Autodesk Fusion 360 part; units mm, degrees
sketch "Sketch1" plane through (0, 0, 0) normal (0, 1, 0) x (1, 0, 0)
  line L0 (1.775, -3.0744) -> (3.55, 0)
  line L1 (3.55, 0) -> (1.775, 3.0744)
  line L2 (1.775, 3.0744) -> (-1.775, 3.0744)
  line L3 (-1.775, 3.0744) -> (-3.55, 0)
  line L4 (-3.55, 0) -> (-1.775, -3.0744)
  line L5 (-1.775, -3.0744) -> (1.775, -3.0744)
  circle A0 centre (0, 0) radius 3.55
  dimension "d6" = 3.55
  dimension "d8" = 7.1
extrude "Extrude1" add sketch "Sketch1" along normal blind 190
sketch "Sketch2" plane through (0, 0, 0) normal (0, 0, 1) x (1, 0, 0)
  line L0 (0, 190) -> (0, 205.8333)
  line L1 (0, 205.8333) -> (3.5149, 190)
  line L2 (0, 190) -> (3.5149, 190)
  dimension "d11" = 15.8333
revolve "Revolve1" add sketch "Sketch2" angle 360 about axis through (0, 190, 0) along (0, 1, 0)
extrude "Extrude2" cut sketch "Sketch1" along normal blind 205 contours L5 A0 | L0 A0 | L1 A0 | L4 A0 | L2 A0 | L3 A0
sketch "Sketch3" plane through (0, 0, 0) normal (1, 0, 0) x (0, 1, 0)
extrude "Extrude3" add sketch "Sketch1" against normal blind 11.7
equation "width = 7.1 mm"
equation "tip_diameter = 2.4 mm"
equation "eraser_holder_height = 11.7 mm"
equation "eraser_height = 4.7 mm"
equation "height = 190 mm"
equation "d6 = width / 2"
equation "d8 = width"
equation "d9 = height"
equation "d11 = height / 12"
equation "d15 = eraser_holder_height * -1"
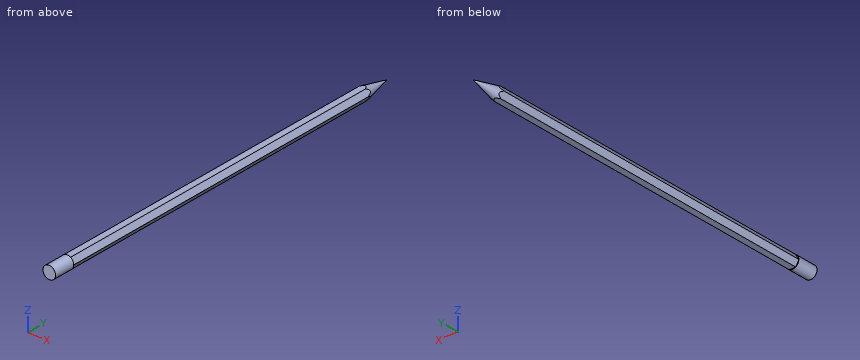
Could you check a few things on this model? Use its own coordinates, in mm. Coordinates: 2 decimals unless noted, no trailing zeros. Write each loop counter-clockwise with the first axis right and the second up, starting at its lowest first coordinate (ties: lowest second). Pieces come first, ordered by that corner, then holes. Notation, with made-up numbers: (40, 30.5) -> (82, 30.5) arc R25 cw to (82, 69.5) -> close; hole circle Ø4 at (24, 0.25). An arc over 180 degrees is marked (long way). One line per question, with ' | ' between items. Start each with the question number.
1. Will these pins go through, and if not, where does the flat tip stop? P1, Ø0.9, axis at x = -3, z = 2, coming from the +Y side; P2, Ø3, axis at x = 0, y = 94, coming from the -Z side; P3, Ø2, axis at x = -0.5, y = 38.5, coming from the +Z side.
2. Please list where these lines run through material, in increasing order: line 1 along Z through (x, y) = (-1.25, 117); line 2 along X through (y, z) = (95, -1); line 3 along Y through (x, z) = (2.25, -2.5).
3. If we section it at A-A (y = 59.5): Please give me the cut outline in (x, z) (3 decimals), and give its area (3 significant figures).
Return value:
1) P1: stops at y = 0 | P2: stops at z = -3.07 | P3: stops at z = 3.07
2) line 1: z = -3.07 to 3.07 | line 2: x = -2.97 to 2.97 | line 3: y = -11.7 to 0
3) outline: (-3.55, 0) -> (-1.775, -3.074) -> (1.775, -3.074) -> (3.55, 0) -> (1.775, 3.074) -> (-1.775, 3.074) -> close | area: 32.7 mm²
